Verification items for the finished model (mm, model axes). A direction names the side the tool comes from. Round coordinates to 2 decimals unless told otherwise and drop trailing zeros. Loops run counter-clockwise (first coordinate to the right, second up) from the corner with the lowest first, then second, coordinate; pieces in that order, holes last. Notation, with made-up numbers: (58, 7.5) - (70, 7.5) arc R13 ccw to (70, 23.5) - close; hole circle Ø11 at (60, 75.25). An arc over 180 degrees is marked (long way). Use CSV: the item, a comma, the result in double quotes.
```python
from build123d import *

# Parameters (mm, degrees)
F0_W          = 76.2
F0_H          = 127
F0_W_2        = 63.5000020266
F0_H_2        = 114.3000020266
F1_DEPTH      = 346.075
F2_R          = 25.4
F3_DEPTH      = 19.05
F5_DEPTH      = 38.1
F5_DEPTH_BACK = 38.1
F6_R          = 15.875
F7_DEPTH      = 50.8


with BuildPart() as f1:
    # F0 (on Right) → F1 (new body, symmetric)
    with BuildSketch(Plane.YZ):
        Rectangle(F0_W, F0_H)
        Rectangle(F0_W_2, F0_H_2, mode=Mode.SUBTRACT)
    extrude(amount=F1_DEPTH, both=True)

    # F2 (on face) → F3 (join)
    with BuildSketch(Plane(origin=(0, 0, -63.5), x_dir=(1, 0, 0), z_dir=(0, 0, -1))):
        with Locations((-307.975, 0)):
            Circle(F2_R)
        with Locations((307.975, 0)):
            Circle(F2_R)
    extrude(amount=F3_DEPTH)

    # F4 (on Front) → F5 (join, two sides)
    with BuildSketch(Plane.XZ) as f5_sk:
        Polygon((-273.05, 75.4103416036), (-317.5, 63.5), (-273.05, 63.5), (-269.8586335857, 63.5), align=None)
        Polygon((269.8586335857, 63.5), (273.05, 63.5), (317.5, 63.5), (273.05, 75.4103416036), align=None)
    extrude(amount=-F5_DEPTH)
    extrude(f5_sk.sketch, amount=F5_DEPTH_BACK)

    # F6 (on face) → F7 (join)
    with BuildSketch(Plane(origin=(0, 0, -82.55), x_dir=(1, 0, 0), z_dir=(0, 0, -1))):
        with Locations((-307.975, 0)):
            Circle(F6_R)
    extrude(amount=F7_DEPTH)

    # F8: F1 across plane


with BuildPart() as f1_1:
    add(f1.part)
    add(f1.part.mirror(Plane.YZ))


solid = f1_1.part
```
1) Mould release check, pull along Y, two halves, no side actions. Record for faces 1 (the face through (5, 31.75, -1)), 2 (the face through (5, 38.1, 5)), 3 (the face through (-332, -1, 63.5)): +Y half, -Y half, draft (parallel to the pull), parting line (faces both ways), or undercut.
Returned:
face 1,"undercut"
face 2,"+Y half"
face 3,"draft"
2) Access from +Z, -Z, +X, -X, +Y, -Y to the whole of each face (thin tool, end or side, straight path). Record for faces 4 (the face through (332, -1, 63.5)), 5 (the face through (4, -1, 63.5)), 6 (the face through (5, -31.75, -1)), 7 (the face through (-320, 11, -82.55)).
Returned:
face 4,"+Z, +X, +Y, -Y"
face 5,"+Z, +Y, -Y"
face 6,"+X, -X"
face 7,"-Z"
3) Gauge pin test, flat ends, axial feed: pin 1 Ø10 at (x, y) = (-132.5, 21) entering from +Z; pin 2 Ø12 at (x, y) = (-40.5, 4.5) entering from -Z. Record the tip position at first contact, or that the pin passes through.
Returned:
pin 1,"stops at z = 63.5"
pin 2,"stops at z = -63.5"
4) Thickness scan on probe 1 along Z at (x, y) = (-14.5, 7.5); probe 2 along Y at (x, z) = (-70, 16.5); probe 3 along Z at (x, y) = (-318, -16). Record the ranges inside material, lowest first. Write a range as [from, to].
Returned:
probe 1,"z = [-63.5, -57.15], [57.15, 63.5]"
probe 2,"y = [-38.1, -31.75], [31.75, 38.1]"
probe 3,"z = [-82.55, -57.15], [57.15, 63.5]"
5) Cross-section at C-C, the plane x = 95.5. Record the cut outline in (y, z), then the cut area to 3 significant figures.
Returned:
outline,"(-38.1, -63.5) - (38.1, -63.5) - (38.1, 63.5) - (-38.1, 63.5) - close; hole (-31.75, -57.15) - (31.75, -57.15) - (31.75, 57.15) - (-31.75, 57.15) - close"
area,"2,420 mm²"
6) Cross-section at A-A, the plane z = 34.5. Record the cut outline in (x, y) (3 decimals).
Returned:
outline,"(-346.075, -38.1) - (346.075, -38.1) - (346.075, -31.75) - (-346.075, -31.75) - close; (-346.075, 31.75) - (346.075, 31.75) - (346.075, 38.1) - (-346.075, 38.1) - close"
